The listing builds one solid part. Answer for the finished solid, in the listing's coordinates (mm). Face numbers are marked on the shaded views. A direction names the side the tool comes from. Coordinates: 2 decimals unless noted, no trailing zeros. Write each loop counter-clockwise with the first axis right and the second up, starting at its lowest first coordinate (ties: lowest second). Pieces come first, ordered by that corner, then holes. Notation, with made-up numbers: M 82,74 L 100,74 A21 cw 100,90 Z; hole C -11.75,28.25 d10. An arc over 180 degrees is marked long. Put each result on its own line as item: value. Start each with the question number.
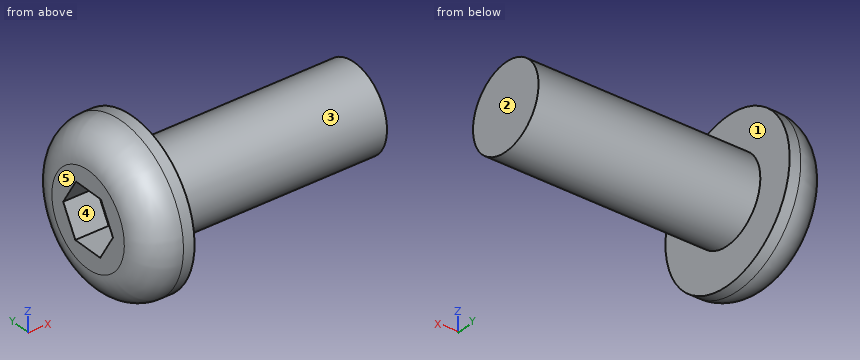
```python
from build123d import *

# Parameters (mm, degrees)
SKETCH1_R           = 4.572
BOSS_EXTRUDE1_DEPTH = 2.54
SKETCH2_R           = 2.413
BOSS_EXTRUDE2_DEPTH = 12.7
FILLET1_R           = 1.905
CUT_EXTRUDE1_DEPTH  = 1.905


with BuildPart() as part:
    # Sketch1 → Boss-Extrude1 (new body)
    with BuildSketch(Plane(origin=(0, 0, 0), x_dir=(0, 0, -1), z_dir=(1, 0, 0))):
        Circle(SKETCH1_R)
    extrude(amount=BOSS_EXTRUDE1_DEPTH)

    # Sketch2 → Boss-Extrude2 (add)
    with BuildSketch(Plane(origin=(2.54, 0, 0), x_dir=(0, 0, -1), z_dir=(1, 0, 0))):
        Circle(SKETCH2_R)
    extrude(amount=BOSS_EXTRUDE2_DEPTH)

    # Fillet1
    fillet1_edges = [part.edges().sort_by_distance(p)[0] for p in [
        (0, 0, 4.572),
    ]]
    fillet(fillet1_edges, radius=FILLET1_R)

    # Sketch3 → Cut-Extrude1 (cut)
    with BuildSketch(Plane.ZY):
        Polygon((1.573613406, -0.940185716), (1.601031418, 0.892696328), (0.027418011, 1.832882044), (-1.573613406, 0.940185716), (-1.601031418, -0.892696328), (-0.027418011, -1.832882044), align=None)
    extrude(amount=-CUT_EXTRUDE1_DEPTH, mode=Mode.SUBTRACT)


solid = part.part
```
1) A cutting plane is placed at B-B on y = 0. Write down the section's boundary in (x, z) (3 decimals).
2) For the marked faces 1 and 2, determine the directions among +Z, -Z, +X, -X, +Y, -Y from which every point of the face is accessible in a straight line to the end or side of a thin tool.
3) Determine the mould class of the marked faces 3, 4 and 5 for opening direction Y: +Y half, -Y half, draft (parallel to the pull), parting line (faces both ways), or undercut.
4) A cutting plane is placed at C-C on x = 7.75. Write down the section's boundary in (y, z).
5) A cutting plane is placed at A-A on x = 2.25. Write down the section's boundary in (y, z), then the cut area to 3 significant figures.
6) Straight lines are drawn through the part: probe 1 along X at (y, z) = (0.5, 2.75); probe 2 along X at (y, z) = (-0.5, -1.25) (3 decimals); probe 3 along Z at (x, y) = (12.5, 1). For each, find the intervals that lie inside material, in ascending order.
7) Given pin 1 Ø4 at (x, y) = (6.5, -1) entering from +Z; pin 2 Ø1 at (y, z) = (3, 2.5) entering from -X; pin 3 Ø1.6 at (y, z) = (0, -0.5) entering from -X (3 decimals), each flat-ended and moving along its own axis, determine where each tip first touches the part or whether it passes through.
Answers follow:
1. outline: M 0,-2.667 A1.905 ccw 1.905,-4.572 L 2.54,-4.572 L 2.54,-2.413 L 15.24,-2.413 L 15.24,2.413 L 2.54,2.413 L 2.54,4.572 L 1.905,4.572 A1.905 ccw 0,2.667 L 0,1.588 L 1.905,1.588 L 1.905,-1.588 L 0,-1.588 Z
2. face 1: +X
2. face 2: +Z, -Z, +X, +Y, -Y
3. face 3: parting line
3. face 4: undercut
3. face 5: draft
4. outline: C 0,0 d4.83
5. outline: C 0,0 d9.14
5. area: 65.7 mm²
6. probe 1: x = 0 to 2.54
6. probe 2: x = 1.905 to 15.24
6. probe 3: z = -2.2 to 2.2
7. pin 1: stops at z = 2.41
7. pin 2: stops at x = 0.15
7. pin 3: stops at x = 1.905
